Source: CAD feature listing. Evaluate the final solid. Frame: model axes, mm. Give positions to 0.01 mm unless a question says otherwise; leave off trailing zeros. One line per question, with ' | ' between items. Start each with the question number.
from build123d import *

# Parameters (mm, degrees)
BOSS_EXTRUDE1_DEPTH = 3


with BuildPart() as part:
    # Model → Boss-Extrude1 (new body)
    with BuildSketch(Plane.XY):
        with BuildLine():
            Line((1159.8, 315.682652611), (1159.8, 268.452661621))
            Line((1159.8, 268.452661621), (1130.6, 268.452661621))
            Line((1130.6, 268.452661621), (1130.6, 288.450029928))
            ThreePointArc((1130.6, 288.450029928), (1099.799999997, 258.052661621), (1130.6, 227.655293314))
            Line((1130.6, 227.655293314), (1130.6, 247.652661621))
            Line((1130.6, 247.652661621), (1159.8, 247.652661621))
            Line((1159.8, 247.652661621), (1159.8, 200.422661621))
            Line((1159.8, 200.422661621), (1051.901037795, 200.422661621))
            Line((1051.901037795, 200.422661621), (1051.901037795, 245.979700014))
            Line((1051.901037795, 245.979700014), (1048.901037796, 245.979700014))
            Line((1048.901037796, 245.979700014), (1048.901037796, 200.422661621))
            Line((1048.901037796, 200.422661621), (892.901037795, 200.422661621))
            Line((892.901037795, 200.422661621), (892.901037795, 245.979700014))
            Line((892.901037795, 245.979700014), (889.901037795, 245.979700014))
            Line((889.901037795, 245.979700014), (889.901037795, 200.422661621))
            Line((889.901037795, 200.422661621), (733.901037795, 200.422661621))
            Line((733.901037795, 200.422661621), (733.901037795, 245.979700014))
            Line((733.901037795, 245.979700014), (730.901037795, 245.979700014))
            Line((730.901037795, 245.979700014), (730.901037795, 200.422661621))
            Line((730.901037795, 200.422661621), (574.901037795, 200.422661621))
            Line((574.901037795, 200.422661621), (574.901037795, 245.979700014))
            Line((574.901037795, 245.979700014), (571.901037795, 245.979700014))
            Line((571.901037795, 245.979700014), (571.901037795, 200.422661621))
            Line((571.901037795, 200.422661621), (415.901037795, 200.422661621))
            Line((415.901037795, 200.422661621), (415.901037795, 245.979700014))
            Line((415.901037795, 245.979700014), (412.901037795, 245.979700014))
            Line((412.901037795, 245.979700014), (412.901037795, 200.422661621))
            Line((412.901037795, 200.422661621), (256.901037795, 200.422661621))
            Line((256.901037795, 200.422661621), (256.901037795, 245.979700014))
            Line((256.901037795, 245.979700014), (253.901037796, 245.979700014))
            Line((253.901037796, 245.979700014), (253.901037796, 200.422661621))
            Line((253.901037796, 200.422661621), (97.901037796, 200.422661621))
            Line((97.901037796, 200.422661621), (97.901037796, 245.979700014))
            Line((97.901037796, 245.979700014), (94.901037796, 245.979700014))
            Line((94.901037796, 245.979700014), (94.901037796, 315.441313757))
            add(Edge.make_bspline(
                [(247.229949675, 319.88819474), (196.438413442, 319.129990608), (145.658637693, 317.812733824), (94.901037796, 315.441313757)],
                knots=[0, 0, 0, 0, 1, 1, 1, 1], degree=3))
            add(Edge.make_bspline(
                [(247.229949675, 319.88819474), (247.232310837, 319.888229986), (247.234672013, 319.888265232), (247.237033201, 319.888300477)],
                knots=[0.554606396, 0.554606396, 0.554606396, 0.554606396, 0.554611125, 0.554611125, 0.554611125, 0.554611125], degree=3))
            add(Edge.make_bspline(
                [(1159.8, 315.682652611), (855.607338384, 318.03324125), (551.339710355, 324.427563161), (247.237033201, 319.888300477)],
                knots=[0, 0, 0, 0, 1, 1, 1, 1], degree=3))
        make_face()
    extrude(amount=BOSS_EXTRUDE1_DEPTH)


solid = part.part
Item 1: Pin query (flat end, axial travel): pin 1 Ø0.9 at (x, z) = (890.5, 1.5) entering from -Y; pin 2 Ø0.9 at (y, z) = (225, 1) entering from -X. Return the tip coordinate at first contact, or that it passes through.
Item 2: Mould query, pull axis Y, two halves, no side actions, for faces 1 (the flat face through (635, 263, 3)), 2 (the cylindrical face through (1099.807, 258.727, 1.479)). Classes: pulls with the +Y half, pulls with the -Y half, needs draft (parallel to the pull), parting line crosses it, or undercut.
Item 3: Line query: line 1 (X direction, y = 282.5, z = 0.2); line 2 (X direction, y = 285, z = 2.6); line 3 (Y direction, x = 763.5, z = 0.25). Output: solid intervals per line, ascending.
Results are:
1) pin 1: stops at y = 245.98 | pin 2: stops at x = 97.9
2) face 1: needs draft | face 2: undercut
3) line 1: x = 94.9 to 1112.13, 1130.6 to 1159.8 | line 2: x = 94.9 to 1116.13, 1130.6 to 1159.8 | line 3: y = 200.42 to 319.81
